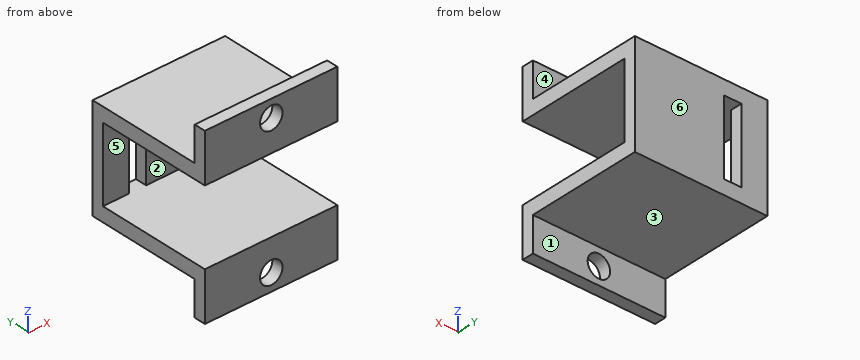
```python
from build123d import *

# Parameters (mm, degrees)
ESQUISSE1_W             = 23
ESQUISSE1_H             = 30
BOSS_EXTRU_1_DEPTH      = 22
ESQUISSE2_W             = 23
ESQUISSE2_H             = 6
ENL_V_MAT_EXTRU_1_DEPTH = 20
D_GAGEMENT_M3_51_D      = 3.9
D_GAGEMENT_M3_51_DEPTH  = 5
D_GAGEMENT_M3_51_TIP    = 1.171678207
ESQUISSE5_W             = 3
ESQUISSE5_H             = 13
ENL_V_MAT_EXTRU_2_DEPTH = 23
ESQUISSE6_W             = 24.5
ESQUISSE6_H             = 13
ENL_V_MAT_EXTRU_3_DEPTH = 20


with BuildPart() as part:
    # Esquisse1 → Boss.-Extru.1 (new body)
    with BuildSketch(Plane(origin=(0, 0, 0), x_dir=(1, 0, 0), z_dir=(0, 1, 0))):
        with Locations((11.5, 15)):
            Rectangle(ESQUISSE1_W, ESQUISSE1_H)
    extrude(amount=BOSS_EXTRU_1_DEPTH)

    # Esquisse2 → Enlèv. mat.-Extru.1 (cut)
    with BuildSketch(Plane(origin=(0, 22, 0), x_dir=(1, 0, 0), z_dir=(0, 1, 0))):
        with Locations((11.5, 27)):
            Rectangle(ESQUISSE2_W, ESQUISSE2_H)
        with Locations((11.5, 3)):
            Rectangle(ESQUISSE2_W, ESQUISSE2_H)
    extrude(amount=-ENL_V_MAT_EXTRU_1_DEPTH, mode=Mode.SUBTRACT)

    # Dégagement M3.51
    with Locations(Plane(origin=(0, 2, 0), x_dir=(1, 0, 0), z_dir=(0, 1, 0))):
        with Locations((11.534470398, 27), (11.534470398, 3)):
            Hole(D_GAGEMENT_M3_51_D / 2, depth=D_GAGEMENT_M3_51_DEPTH)
            with Locations((0, 0, -(D_GAGEMENT_M3_51_DEPTH + D_GAGEMENT_M3_51_TIP / 2))):  # 118° drill point
                Cone(0, D_GAGEMENT_M3_51_D / 2, D_GAGEMENT_M3_51_TIP, mode=Mode.SUBTRACT)

    # Esquisse5 → Enlèv. mat.-Extru.2 (cut, through all)
    with BuildSketch(Plane(origin=(0, 22, 0), x_dir=(1, 0, 0), z_dir=(0, 1, 0))):
        with Locations((6, 15)):
            Rectangle(ESQUISSE5_W, ESQUISSE5_H)
    extrude(amount=-ENL_V_MAT_EXTRU_2_DEPTH, mode=Mode.SUBTRACT)

    # Esquisse6 → Enlèv. mat.-Extru.3 (cut)
    with BuildSketch(Plane.XZ):
        with Locations((12.25, -15)):
            Rectangle(ESQUISSE6_W, ESQUISSE6_H)
    extrude(amount=-ENL_V_MAT_EXTRU_3_DEPTH, mode=Mode.SUBTRACT)


solid = part.part
```
Model file for the job. Use its own axes, mm. Face numbers are marked on the shaded views. A direction names the side the tool comes from. Round coordinates to 2 decimals unless told otherwise and drop trailing zeros. Write each loop counter-clockwise with the first axis right and the second up, starting at its lowest first coordinate (ties: lowest second). Pieces come first, ordered by that corner, then holes. Notation, with made-up numbers: M 3,-20.5 L 61,-20.5 A9 ccw 61,-16.5 Z; hole C -38,40.5 d3. An arc over 180 degrees is marked long. Put each result on its own line as item: value.
Item 1: Cut at C-C (y = 9). List the corners of the cut face in (x, z), and give its area (3 significant figures).
Responses:
outline: M 0,-24 L 23,-24 L 23,-21.5 L 0,-21.5 Z; M 0,-8.5 L 23,-8.5 L 23,-6 L 0,-6 Z
area: 115 mm²
Item 2: Mould opens along Z. For the marked faces 1, 2 and 3 say: +Z half, -Z half, draft (parallel to the pull), parting line (faces both ways), or undercut.
Responses:
face 1: draft
face 2: undercut
face 3: -Z half
Item 3: Cut at A-A (y = 1.5). List the corners of the cut face in (x, z), and give its area (3 significant figures).
Responses:
outline: M 0,-30 L 23,-30 L 23,-21.5 L 0,-21.5 Z; M 0,-8.5 L 23,-8.5 L 23,0 L 0,0 Z; hole C 11.53,-27 d3.9; hole C 11.53,-3 d3.9
area: 367 mm²
Item 4: Tool access for the marked faces 4, 5 and 6: list every direction of +Z, -Z, +X, -X, +Y, -Y with a clear straight run to the whole face (end or side of a thin tool).
Responses:
face 4: +Z, +X, -X, +Y
face 5: +X, -X, -Y
face 6: +Z, -Z, +X, -X, +Y
Item 5: Flat gauge pins, fed straight in: P1, Ø1.5, axis at x = 16.5, y = 5, coming from the +Z side; P2, Ø6.5, axis at x = 7.5, z = -4, coming from the +Y side; P3, Ø10, axis at x = 16.5, y = 18.5, coming from the -Z side; P4, Ø5, axis at x = 1.5, z = -12, coming from the -Y side. Where does each tip first touch, or does it go through?
Responses:
P1: z = -6
P2: y = 22
P3: z = -24
P4: y = 20
Item 6: Cut at B-B (z = -11.75). List the corners of the cut face in (x, y).
Responses:
outline: M 0,20 L 4.5,20 L 4.5,22 L 0,22 Z; M 7.5,20 L 23,20 L 23,22 L 7.5,22 Z
Item 7: Probe L1, parallel to Z at x = 3.5, y = 18; L2, parallel to X at y = 1.4, z = -27; L3, parallel to Z at x = 18.25, y = 1.75. List the from-to ranges inside material, lowest first. Write a range as from..to.
Responses:
L1: -24..-21.5, -8.5..-6
L2: 0..9.58, 13.48..23
L3: -30..-21.5, -8.5..0
Item 8: Cut at D-D (x = 2.75). List the corners of the cut face in (y, z), and give its area (3 significant figures).
Responses:
outline: M 0,-30 L 2,-30 L 2,-24 L 22,-24 L 22,-6 L 2,-6 L 2,0 L 0,0 L 0,-8.5 L 20,-8.5 L 20,-21.5 L 0,-21.5 Z
area: 160 mm²
